The listing builds one solid part. Answer for the finished solid, in the listing's coordinates (mm). A direction names the side the tool comes from. Coordinates: 2 decimals unless noted, no trailing zeros. Order: outer loops, then holes, each group sorted by start corner. A loop starts at its lowest first (then second) coordinate and runs counter-clockwise, first axis right, second up.
```python
from build123d import *

# Parameters (mm, degrees)
BOSS_EXTRUDE1_DEPTH = 1.5
SKETCH2_W           = 3
SKETCH2_H           = 10
BOSS_EXTRUDE2_DEPTH = 15
SKETCH3_W           = 10
SKETCH3_H           = 2
BOSS_EXTRUDE3_DEPTH = 12


with BuildPart() as part:
    # Sketch1 → Boss-Extrude1 (new body)
    with BuildSketch(Plane(origin=(0, 0, 0), x_dir=(1, 0, 0), z_dir=(0, 1, 0))):
        Polygon((-10.25315493, 4.457893448), (-22.27397021, -7.562921833), (-15.202902398, -14.633989644), (-6.111019306, -5.542106552), (12.74684507, -5.542106552), (12.74684507, 4.457893448), align=None)
    extrude(amount=BOSS_EXTRUDE1_DEPTH)

    # Sketch2 → Boss-Extrude2 (add)
    with BuildSketch(Plane.XZ):
        with Locations((11.24684507, 0.542106552)):
            Rectangle(SKETCH2_W, SKETCH2_H)
    extrude(amount=BOSS_EXTRUDE2_DEPTH)

    # Sketch3 → Boss-Extrude3 (add)
    with BuildSketch(Plane.ZY.offset(-9.74684507)):
        with Locations((0.542106552, -14)):
            Rectangle(SKETCH3_W, SKETCH3_H)
    extrude(amount=BOSS_EXTRUDE3_DEPTH)


solid = part.part
```
(1) For faces 5 (the face through (-2.253, -14, 0)), 6 (the face through (4, -13, 0)), 7 (the face through (10, -7, 5.542)), 8 (the face through (12.747, -7, 0)), 9 (the face through (10, -7, -4.458)), determine the directions among +Z, -Z, +X, -X, +Y, -Y from which every point of the face is accessible in a straight line to the end or side of a thin tool.
(2) Find section A-A (x = -1). Write down the section's boundary in (y, z).
(3) Consider line 1 (Y direction, x = -0.5, z = 4.75); line 2 (X direction, y = -1.75, z = 2.75); line 3 (Y direction, x = -3.5, z = -2.25). Determine where each line is inside the solid, lowest interval first.
(4) Each of these flat-tipped pins is pushed along its axis until it touches: pin 1 Ø6 at (x, y) = (9, -13.5) entering from +Z; pin 2 Ø3 at (y, z) = (-4.5, 2) entering from -X; pin 3 Ø9.5 at (x, z) = (-7.5, 8) entering from -Y. Where does it stop, or does it pass through?
(5) Find section C-C (z = 1.25). Write down the section's boundary in (x, y), and give its area (3 significant figures).
(6) The mould has two halves that part along Y. Classify faces 1 (the face through (-16.18, 0.74, 1.47)), 2 (the face through (5, -15, 0)), 3 (the face through (-5, 1.5, 3)), 4 (the face through (9.747, -6, 0)): released by +Y, released by -Y, zero draft, split by the parting line, or undercut.
(7) Find section D-D (x = -5). Write down the section's boundary in (y, z), and give its area (3 significant figures).
(8) Find section B-B (y = 0.5). Write down the section's boundary in (x, z).
Findings below:
1. face 5: +Z, -Z, -X, -Y
1. face 6: +Z, -Z, -X
1. face 7: +Z, +X, +Y, -Y
1. face 8: +Z, -Z, +X, +Y, -Y
1. face 9: -Z, +X, -X, +Y, -Y
2. outline: (-15, -4.46) - (-13, -4.46) - (-13, 5.54) - (-15, 5.54) - close; (0, -4.46) - (1.5, -4.46) - (1.5, 5.54) - (0, 5.54) - close
3. line 1: y = -15 to -13, 0 to 1.5
3. line 2: x = 9.75 to 12.75
3. line 3: y = 0 to 1.5
4. pin 1: stops at z = 5.54
4. pin 2: stops at x = 9.75
4. pin 3: stops at y = 0
5. outline: (-15.96, 0) - (9.75, 0) - (9.75, -13) - (-2.25, -13) - (-2.25, -15) - (12.75, -15) - (12.75, 1.5) - (-15.96, 1.5) - close
5. area: 112 mm2
6. face 1: zero draft
6. face 2: released by -Y
6. face 3: released by +Y
6. face 4: undercut
7. outline: (0, -4.46) - (1.5, -4.46) - (1.5, 5.54) - (0, 5.54) - close
7. area: 15.0 mm2
8. outline: (-22.27, 7.56) - (-10.25, -4.46) - (12.75, -4.46) - (12.75, 5.54) - (-6.11, 5.54) - (-15.2, 14.63) - close
